```python
from build123d import *

# Parameters (mm, degrees)
CUT_EXTRUDE1_DEPTH      = 17
CUT_EXTRUDE1_DEPTH_BACK = 17


with BuildPart() as part:
    # Sketch1 → Revolve1 (revolve)
    with BuildSketch(Plane(origin=(0, 0, 0), x_dir=(0, 0, -1), z_dir=(1, 0, 0)), mode=Mode.PRIVATE) as revolve1_sk:
        Polygon((-35.8, 0), (-35.8, 9.717157288), (-35.517157288, 10), (116.333333333, 10), (116.333333333, 25), (133, 25), (133, 0), align=None)
    revolve(revolve1_sk.sketch.rotate(Axis((0, 0, -133), (0, 0, 1)), 270), axis=Axis((0, 0, -133), (0, 0, 1)))

    # Sketch2 → Cut-Extrude1 (cut, two sides: drawn at the far end of the back side and taken through both)
    with BuildSketch(Plane(origin=(0, 0, 0), x_dir=(1, 0, 0), z_dir=(0, 1, 0)).offset(-CUT_EXTRUDE1_DEPTH_BACK)):
        Polygon((-17, -61.8), (17, -61.8), (17, -27.8), (8.5, -27.8), (8.5, -43.8), (-8.5, -43.8), (-8.5, -27.8), (-17, -27.8), align=None)
    extrude(amount=CUT_EXTRUDE1_DEPTH + CUT_EXTRUDE1_DEPTH_BACK, mode=Mode.SUBTRACT)

    # Sketch3 → Revolve2 (revolve)
    with BuildSketch(Plane(origin=(0, 0, 0), x_dir=(0, 0, -1), z_dir=(1, 0, 0)), mode=Mode.PRIVATE) as revolve2_sk:
        with BuildLine():
            Line((-67.8, 0), (-67.8, 7.08))
            Line((-67.8, 7.08), (-66.88, 8))
            Line((-66.88, 8), (-41.28485129, 8))
            Line((-41.28485129, 8), (-38.524269872, 6.995230534))
            ThreePointArc((-38.524269872, 6.995230534), (-38.397990898, 6.961394185), (-38.267754764, 6.95))
            Line((-38.267754764, 6.95), (-36.55, 6.95))
            ThreePointArc((-36.55, 6.95), (-36.019669914, 7.169669914), (-35.8, 7.7))
            Line((-35.8, 7.7), (-35.05, 7.7))
            Line((-35.05, 7.7), (-35.05, 0))
            Line((-35.05, 0), (-67.8, 0))
        make_face()
    revolve(revolve2_sk.sketch.rotate(Axis((0, 0, 35.05), (0, 0, 1)), 270), axis=Axis((0, 0, 35.05), (0, 0, 1)))


solid = part.part
```
For this review, take the finished solid that the model builds, in its own axes (mm). A direction names the side the tool comes from. Round coordinates to 2 decimals unless told otherwise and drop trailing zeros. Write each loop counter-clockwise with the first axis right and the second up, starting at its lowest first coordinate (ties: lowest second). Pieces come first, ordered by that corner, then holes. Notation, with made-up numbers: (42, 37.5) -> (76, 37.5) arc R20 cw to (76, 69.5) -> close; hole circle Ø7 at (81.25, 75.5). An arc over 180 degrees is marked (long way). One line per question, with ' | ' between items. Start each with the question number.
1) Machinability: for faces 5 (the flat face through (-8.5, 0, 32)), 6 (the cylindrical face through (-2.17, -9.76, -41.47)), 7 (the flat face through (8.5, 0, 32)), 8 (the flat face through (0, -8, 35.8)), which of the approach directions +Z, -Z, +X, -X, +Y, -Y give a long, thin tool a straight path to every point of the face, cutting with its end or side? Answer none if there is none.
2) Add section C-C (z = -7). Write out the cut boundary in (x, y), and give its area (3 significant figures).
3) For pin 1 Ø8 at (x, z) = (12, -61) entering from -Y; pin 2 Ø5 at (x, z) = (14.5, -42.5) entering from +Y; pin 3 Ø0.8 at (x, y) = (-9, 0.5) entering from +Z; pin 4 Ø4 at (x, z) = (-1, -106.5) entering from -Y, all flat-tipped, find the tip position at first contact; note any pin that passes through.
4) Add section D-D (y = 12). Write out the cut boundary in (x, z).
5) Add section B-B (y = 0). Write out the cut boundary in (x, z).
6) Add section A-A (x = 0). Write out the cut boundary in (y, z).
7) Wall thickness on line 1 along Z through (x, y) = (13.5, -15.5); line 2 along Y through (x, z) = (0.5, 46.5); line 3 along Z through (x, y) = (-9, 2): over which ranges is each line inside the solid? List them lowest first.
8) Mouldability with a two-part tool opening along Z and no side actions: class faces 1 (the conical face through (-0.9, 7, 38.7)), 2 (the cylindrical face through (-1.73, -7.81, 53.9)), 3 (the flat face through (0, 0, 67.8)), 4 (the flat face through (0, 0, -133)) as +Z half, -Z half, draft (parallel to the pull), parting line (faces both ways), or undercut.
Reported:
1) face 5: +Z, -X, +Y, -Y | face 6: +Z | face 7: +Z, +X, +Y, -Y | face 8: none
2) outline: circle Ø20 at (0, 0) | area: 314 mm²
3) pin 1: stops at y = -6 | pin 2: passes through | pin 3: stops at z = 27.8 | pin 4: stops at y = -10
4) outline: (-21.93, -133) -> (21.93, -133) -> (21.93, -116.33) -> (-21.93, -116.33) -> close
5) outline: (-25, -133) -> (25, -133) -> (25, -116.33) -> (10, -116.33) -> (10, 27.8) -> (8.5, 27.8) -> (8.5, 35.8) -> (7.7, 35.8) arc R0.75 cw to (6.95, 36.55) -> (6.95, 38.27) arc R0.75 cw to (7, 38.52) -> (8, 41.28) -> (8, 66.88) -> (7.08, 67.8) -> (-7.08, 67.8) -> (-8, 66.88) -> (-8, 41.28) -> (-7, 38.52) arc R0.75 cw to (-6.95, 38.27) -> (-6.95, 36.55) arc R0.75 cw to (-7.7, 35.8) -> (-8.5, 35.8) -> (-8.5, 27.8) -> (-10, 27.8) -> (-10, -116.33) -> (-25, -116.33) -> close
6) outline: (-25, -133) -> (25, -133) -> (25, -116.33) -> (10, -116.33) -> (10, 35.52) -> (9.72, 35.8) -> (7.7, 35.8) arc R0.75 cw to (6.95, 36.55) -> (6.95, 38.27) arc R0.75 cw to (7, 38.52) -> (8, 41.28) -> (8, 66.88) -> (7.08, 67.8) -> (-7.08, 67.8) -> (-8, 66.88) -> (-8, 41.28) -> (-7, 38.52) arc R0.75 cw to (-6.95, 38.27) -> (-6.95, 36.55) arc R0.75 cw to (-7.7, 35.8) -> (-9.72, 35.8) -> (-10, 35.52) -> (-10, -116.33) -> (-25, -116.33) -> close
7) line 1: z = -133 to -116.33 | line 2: y = -7.98 to 7.98 | line 3: z = -133 to 27.8
8) face 1: undercut | face 2: draft | face 3: +Z half | face 4: -Z half
